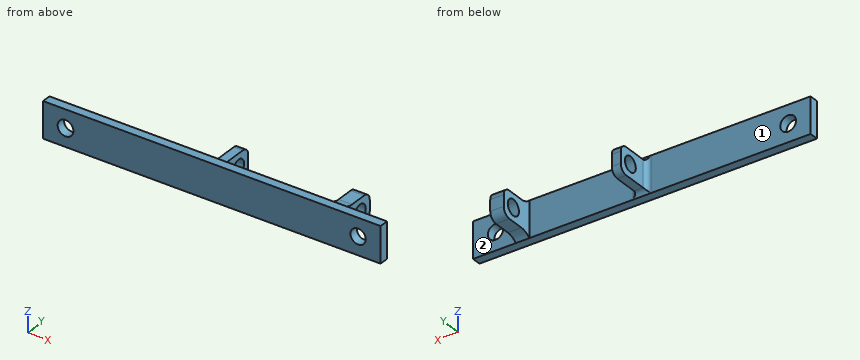
```python
from build123d import *

# Parameters (mm, degrees)
SKETCH_1_W           = 75
SKETCH_1_H           = 8
SKETCH_1_R           = 1.75
SKETCH_1_R_2         = 1.7
EXTRUDE_1_DEPTH      = 2
EXTRUDE_2_DEPTH      = 1
EXTRUDE_2_DEPTH_BACK = 1
SKETCH_2_W           = 6
SKETCH_2_H           = 8
SKETCH_2_R           = 1.7
FILLET_2_R           = 1
FILLET_3_R           = 1.7
SKETCH_3_W           = 6
SKETCH_3_H           = 8
SKETCH_3_R           = 1.75
EXTRUDE_3_DEPTH      = 3
FILLET_6_R           = 1.75
FILLET_7_R           = 3.5


# Some blends are built 0.0001 mm under size
with BuildPart() as part:
    # 草图1 → 凸台-拉伸1 (new body)
    with BuildSketch(Plane(origin=(0, 0, 0), x_dir=(1, 0, 0), z_dir=(0, 1, 0))):
        Rectangle(SKETCH_1_W, SKETCH_1_H)
        with Locations(Location((-32.5, 0, 0), (0, 0, 270))):
            Circle(SKETCH_1_R, mode=Mode.SUBTRACT)
        with Locations(Location((32.5, 0, 0), (0, 0, 270))):
            Circle(SKETCH_1_R_2, mode=Mode.SUBTRACT)
    extrude(amount=EXTRUDE_1_DEPTH)

    # 草图2 → 凸台-拉伸2 (add, two sides: drawn at the far end of the back side and taken through both)
    with BuildSketch(Plane(origin=(0, 0, 0), x_dir=(0, 0, -1), z_dir=(1, 0, 0)).offset(-EXTRUDE_2_DEPTH_BACK)):
        with Locations((0, 6)):
            Rectangle(SKETCH_2_W, SKETCH_2_H)
        with Locations((0, 7)):
            Circle(SKETCH_2_R, mode=Mode.SUBTRACT)
    extrude(amount=EXTRUDE_2_DEPTH + EXTRUDE_2_DEPTH_BACK)

    # 圆角2
    fillet_2_edges = [part.edges().sort_by_distance(p)[0] for p in [
        (0, 2, -3),
        (-1, 2, 0),
        (0, 2, 3),
        (1, 2, 0),
    ]]
    fillet(fillet_2_edges, radius=FILLET_2_R - 0.0001)  # a hair under: the kernel refuses the full size

    # 圆角3
    fillet_3_edges = [part.edges().sort_by_distance(p)[0] for p in [
        (0, 10, -3),
        (0, 10, 3),
    ]]
    fillet(fillet_3_edges, radius=FILLET_3_R)

    # 草图3 → 凸台-拉伸3 (add)
    with BuildSketch(Plane(origin=(28, 0, 0), x_dir=(0, 0, -1), z_dir=(1, 0, 0))):
        with Locations((0, 6)):
            Rectangle(SKETCH_3_W, SKETCH_3_H)
        with Locations((0, 7)):
            Circle(SKETCH_3_R, mode=Mode.SUBTRACT)
    extrude(amount=-EXTRUDE_3_DEPTH)

    # 圆角6
    fillet_6_edges = [part.edges().sort_by_distance(p)[0] for p in [
        (26.5, 10, -3),
        (26.5, 10, 3),
    ]]
    fillet(fillet_6_edges, radius=FILLET_6_R)

    # 圆角7
    # the kernel refuses this fillet: 3.5 mm, written as the material it adds along each edge
    with BuildSketch(Plane(origin=(28, 2, -3), x_dir=(0, 0, -1), z_dir=(-1, 0, 0))) as fillet_7_piece_1:
        with BuildLine():
            CenterArc((3.5, -2.449489743), FILLET_7_R, 135.584691403, 44.415308597)
            Line((0, -2.449489743), (-0.07, -2.449489743))
            Line((-0.07, -2.449489743), (-0.07, 0))
            Line((-0.07, 0), (0, 0.07))
            ThreePointArc((0, 0.07), (0.5, 0.07), (0.95, 0.048989795))
            Line((0.95, 0.048989795), (1, 0))
        make_face()
    extrude(amount=3)
    with BuildSketch(Plane(origin=(28, 2, 3), x_dir=(0, 1, 0), z_dir=(-1, 0, 0))) as fillet_7_piece_2:
        with BuildLine():
            CenterArc((2.449489743, -3.5), FILLET_7_R, 90, 44.415308597)
            Line((0, -1), (-0.048989795, -0.95))
            ThreePointArc((-0.048989795, -0.95), (-0.07, -0.5), (-0.07, 0))
            Line((-0.07, 0), (0, 0.07))
            Line((0, 0.07), (2.449489743, 0.07))
            Line((2.449489743, 0.07), (2.449489743, 0))
        make_face()
    extrude(amount=3)


solid = part.part
```
Model file for the job. Use its own axes, mm. Face numbers are marked on the shaded views. Round coordinates to 2 decimals unless told otherwise and drop trailing zeros. Write each loop counter-clockwise with the first axis right and the second up, starting at its lowest first coordinate (ties: lowest second). Pieces come first, ordered by that corner, then holes. Notation, with made-up numbers: (88, 79) - (95, 79) arc R12 ccw to (95, 94) - close; hole circle Ø6 at (26.25, -39). An arc over 180 degrees is marked (long way). One line per item, written item: value.
(1) Drop flat-ended pins along their axis: P1, Ø2.5, axis at x = 30.5, z = 0.5, coming from the +Y side; P2, Ø4, axis at y = 7, z = 0, coming from the -X side; P3, Ø1.6, axis at x = 0, y = 5.5, coming from the -Z side. Give the stop position or say it passes through.
Values follow:
P1: stops at y = 2
P2: stops at x = -1
P3: stops at z = -3
(2) Cut at C-C, the plane y = 7. Give the cut face in (x, z).
Values follow:
outline: (-1, -3) - (1, -3) - (1, -1.7) - (-1, -1.7) - close; (-1, 1.7) - (1, 1.7) - (1, 3) - (-1, 3) - close; (25, -3) - (28, -3) - (28, -1.75) - (25, -1.75) - close; (25, 1.75) - (28, 1.75) - (28, 3) - (25, 3) - close
(3) Cut at A-A, the plane x = 32.5. Give the cut face in (y, z).
Values follow:
outline: (0, -4) - (2, -4) - (2, -1.7) - (0, -1.7) - close; (0, 1.7) - (2, 1.7) - (2, 4) - (0, 4) - close
(4) Wall check: probe 1 along X at (y, z) = (1.35, 0); probe 2 along Y at (x, z) = (0.5, 0); probe 3 along X at (y, z) = (6.25, -2.5). Give the ranges that are in metal, low to high.
Values follow:
probe 1: x = -37.5 to -34.25, -30.75 to 30.8, 34.2 to 37.5
probe 2: y = 0 to 5.3, 8.7 to 10
probe 3: x = -1 to 1, 25 to 28
(5) Cut at B-B, the plane z = 0. Give the number of separate pieces and of enclosed holes in the cut face, plus the area to 3 significant figures.
Values follow:
separate pieces: 5
enclosed holes: 0
area: 159 mm²
(6) Two-plate mould, pull along X, no slides. Class the marked faces 1 and 2: pulls with the +X half, pulls with the -X half, needs draft (parallel to the pull), parting line crosses it, or undercut.
Values follow:
face 1: needs draft
face 2: needs draft
(7) Cut at D-D, the plane y = 1.25. Give the cut face in (x, z), plus the area to 3 significant figures.
Values follow:
outline: (-37.5, -4) - (37.5, -4) - (37.5, 4) - (-37.5, 4) - close; hole circle Ø3.5 at (-32.5, 0); hole circle Ø3.4 at (32.5, 0)
area: 581 mm²
